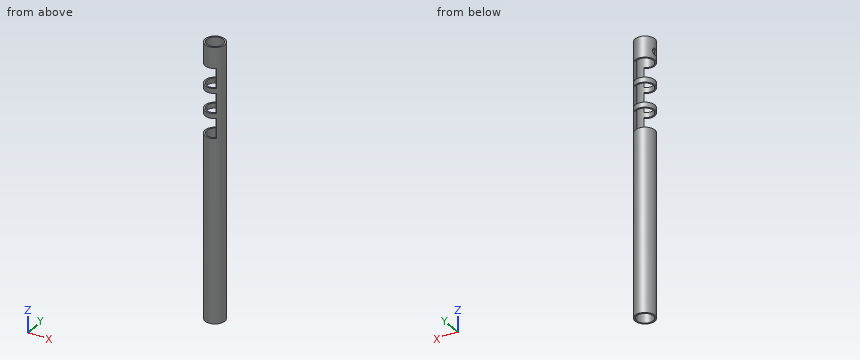
from build123d import *

# Parameters (mm, degrees)
SURFACE_EXTRUDE1_1_DEPTH   = 1.866
SURFACE_TRIM1_TOOL_2_BACK  = 3.327
SURFACE_TRIM1_TOOL_2_DEPTH = 6.654
THICKEN2_T1                = 0.101386
LPATTERN3_COUNT            = 3
LPATTERN3_PITCH            = 1.555
BOSS_EXTRUDE1_DEPTH        = 11.21
BOSS_EXTRUDE2_DEPTH        = 1
SKETCH7_R                  = 0.2
CUT_EXTRUDE2_DEPTH         = 12.244459436


with BuildPart() as body_1:
    # Surface-Extrude1: a surface, the sketch's curves swept straight by 1.866 mm
    with BuildLine(Plane.XY, mode=Mode.PRIVATE) as surface_extrude1_1_path:
        ThreePointArc((0.622, 0), (0, 0.622), (-0.622, 0))
    surface_extrude1_1 = Shell.extrude(surface_extrude1_1_path.wire(), (0 * SURFACE_EXTRUDE1_1_DEPTH, 0 * SURFACE_EXTRUDE1_1_DEPTH, 1 * SURFACE_EXTRUDE1_1_DEPTH))
    # Surface-Trim1 tool: a surface, the sketch's curves swept straight by 6.654 mm
    with BuildLine(Plane(origin=(0, 0, 0), x_dir=(1, 0, 0), z_dir=(0, 1, 0)).offset(-SURFACE_TRIM1_TOOL_2_BACK), mode=Mode.PRIVATE) as surface_trim1_tool_2_path:
        Line((-0.622, -1.555), (0.3932, -1.555))
        Line((0.3932, -1.555), (0.3932, -0.311))
        Line((0.3932, -0.311), (-0.622, -0.311))
    surface_trim1_tool_2 = Shell.extrude(surface_trim1_tool_2_path.wire(), (0 * SURFACE_TRIM1_TOOL_2_DEPTH, 1 * SURFACE_TRIM1_TOOL_2_DEPTH, 0 * SURFACE_TRIM1_TOOL_2_DEPTH))
    # Surface-Trim1: the surface trimmed, the side behind the tool kept
    surface_trim1_3 = split(surface_extrude1_1.faces()[0], bisect_by=surface_trim1_tool_2, keep=Keep.BOTTOM).faces()[0]
    add(Solid.thicken(surface_trim1_3, THICKEN2_T1))


with BuildPart() as lpattern3_1:
    # LPattern3: pattern copy
    add(body_1.part.moved(Location(Vector(0, 0, 1) * (1 * LPATTERN3_PITCH))))


with BuildPart() as lpattern3_2:
    # LPattern3: pattern copy
    add(body_1.part.moved(Location(Vector(0, 0, 1) * (2 * LPATTERN3_PITCH))))


with BuildPart() as body_1_1:
    add(body_1.part)

    # Combine1: read off the stored shape, not the designer's step
    # Combine1: union LPattern3_2, LPattern3_1
    add(lpattern3_2.part)
    add(lpattern3_1.part)

    # Sketch5 → Boss-Extrude1 (add)
    with BuildSketch(Plane(origin=(0, 0, 0), x_dir=(-1, 0, 0), z_dir=(0, 0, -1))):
        with BuildLine():
            Line((-0.622, 0), (-0.520614, 0))
            ThreePointArc((-0.520614, 0), (0, 0.520614), (0.520614, 0))
            Line((0.520614, 0), (0.622, 0))
            ThreePointArc((0.622, 0), (0, 0.622), (-0.622, 0))
        make_face()
    extrude(amount=BOSS_EXTRUDE1_DEPTH)

    # Sketch6 → Boss-Extrude2 (add)
    with BuildSketch(Plane.XY.offset(4.976)):
        with BuildLine():
            Line((-0.622, 0), (-0.520614, 0))
            ThreePointArc((-0.520614, 0), (0, 0.520614), (0.520614, 0))
            Line((0.520614, 0), (0.622, 0))
            ThreePointArc((0.622, 0), (0, 0.622), (-0.622, 0))
        make_face()
    extrude(amount=BOSS_EXTRUDE2_DEPTH)

    # Sketch7 → Cut-Extrude2 (cut, through all)
    with BuildSketch(Plane(origin=(0, 0, 0), x_dir=(0, 0, -1), z_dir=(1, 0, 0))):
        with Locations((-5.165, 0)):
            Circle(SKETCH7_R)
    extrude(amount=-CUT_EXTRUDE2_DEPTH, mode=Mode.SUBTRACT)

    # Mirror1: body 1 across face


with BuildPart() as body_1_2:
    add(body_1_1.part)
    add(body_1_1.part.mirror(Plane(origin=(0.571307, 0, -2.617), x_dir=(0, 0, 1), z_dir=(0, -1, 0))))


solid = body_1_2.part
Check sheet for the modelled part. Datum: model origin and axes. Units: mm. Round coordinates to 2 decimals unless told otherwise and drop trailing zeros. Loops run counter-clockwise (first coordinate to the right, second up) from the corner with the lowest first, then second, coordinate; pieces in that order, holes last. Notation, with made-up numbers: M 48.25,68.25 L 66.25,68.25 A13 cw 66.25,74.25 Z; hole C -20,36 d8. An arc over 180 degrees is marked long. One line per question, with ' | ' between items. Start each with the question number.
Item 1: Section check B-B (z = -4.5). Record the boundary of the cut face in (x, y).
Item 2: Section check C-C (z = 2.25). Record the boundary of the cut face in (x, y).
Item 3: Scan line: probe 1 along X at (y, z) = (0.45, -1.5). Record every from-to range of solid material in increasing order.
Item 4: Section check A-A (x = 0). State how many separate pieces and enclosed holes the cut face has, and give its area (3 significant figures).
Worked out:
1) outline: C 0,0 d1.24; hole C 0,0 d1.04
2) outline: M 0.33,-0.4 L 0.39,-0.48 A0.62 ccw 0.39,0.48 L 0.33,0.4 A0.52 cw Z
3) probe 1: -0.43 to -0.26, 0.26 to 0.43
4) separate pieces: 8 | enclosed holes: 0 | area: 2.73 mm^2
